from build123d import *

# Parameters (mm, degrees)
EXTRUDE_1_DEPTH     = 16
CUT_EXTRUDE_1_DEPTH = 50
EXTRUDE_2_DEPTH     = 28.5
SKETCH_4_R          = 4.5
CUT_EXTRUDE_2_DEPTH = 28.5


with BuildPart() as part:
    # 草图1 → 凸台-拉伸1 (new, symmetric)
    with BuildSketch(Plane.XY):
        with BuildLine():
            Line((-17, 0), (-17, -66.86388681))
            Line((-17, -66.86388681), (-20.5, -66.86388681))
            Line((-20.5, -66.86388681), (-20.5, 0))
            ThreePointArc((-20.5, 0), (0, 20.5), (20.5, 0))
            Line((20.5, 0), (20.5, -66.86388681))
            Line((20.5, -66.86388681), (17, -66.86388681))
            Line((17, -66.86388681), (17, 0))
            ThreePointArc((17, 0), (0, 17), (-17, 0))
        make_face()
    extrude(amount=EXTRUDE_1_DEPTH, both=True)

    # 草图2 → 切除-拉伸1 (cut, symmetric)
    with BuildSketch(Plane(origin=(0, 0, 0), x_dir=(0, 0, -1), z_dir=(1, 0, 0))):
        Polygon((16, -42.748653355), (-16, -38.251346645), (-16, -66.86388681), (16, -66.86388681), align=None)
    extrude(amount=CUT_EXTRUDE_1_DEPTH, both=True, mode=Mode.SUBTRACT)

    # 草图3 → 凸台-拉伸2 (add)
    with BuildSketch(Plane.ZY.offset(20.5)):
        Polygon((-16, -42.748653355), (16, -38.251346645), (16, -34.716950141), (-16, -39.214256851), align=None)
    extrude_2 = extrude(amount=EXTRUDE_2_DEPTH)

    # 镜向1: 凸台-拉伸2 across plane
    add(extrude_2.mirror(Plane(origin=(0, 0, 0), x_dir=(0, 0, 1), z_dir=(1, 0, 0))))

    # 草图4 → 切除-拉伸2 (cut)
    with BuildSketch(Plane(origin=(0, -36.249611102, 5.094550602), x_dir=(1, 0, 0), z_dir=(0, 0.9902680687415715, -0.13917310096005808))):
        with Locations(Location((40.5, 5.144617667, 0), (0, 0, 270))):
            Circle(SKETCH_4_R)
        with BuildLine():
            Line((-36, 7.644617667), (-36, 2.644617667))
            ThreePointArc((-36, 2.644617667), (-40.5, -1.855382333), (-45, 2.644617667))
            Line((-45, 2.644617667), (-45, 7.644617667))
            ThreePointArc((-45, 7.644617667), (-40.5, 12.144617667), (-36, 7.644617667))
        make_face()
    extrude(amount=-CUT_EXTRUDE_2_DEPTH, mode=Mode.SUBTRACT)


solid = part.part
Input: part model. Units: mm. Frame: model coordinates. A direction names the side the tool comes from. Coordinates: 2 decimals unless noted, no trailing zeros. Order: outer loops, then holes, each group sorted by start corner. A loop starts at its lowest first (then second) coordinate and runs counter-clockwise, first axis right, second up. Notation, with made-up numbers: M 51.5,51 L 109.5,51 A35 ccw 109.5,86 Z; hole C 55,-21 d10. An arc over 180 degrees is marked long. Answer in a Markdown table with one row per item.
(1) Contact query for flat-ended pins moving along their axis: pin 1 Ø3 at (y, z) = (-32, -12) entering from -X; pin 2 Ø12 at (y, z) = (13.5, 0) entering from +X; pin 3 Ø5 at (x, z) = (26, -13) entering from +Y. Output: stop coordinate, or through.
Numbers:
| item | result |
|---|---|
| pin 1 | stops at x = -20.5 |
| pin 2 | stops at x = 19.08 |
| pin 3 | stops at y = -38.44 |
(2) Section query C-C, the plane z = 13.5. Output: boundary loops of the cut face in (x, y), plus the area to 3 significant figures.
Numbers:
| item | result |
|---|---|
| outline | M -49,-38.6 L -17,-38.6 L -17,0 A17 cw 17,0 L 17,-38.6 L 49,-38.6 L 49,-35.07 L 20.5,-35.07 L 20.5,0 A20.5 ccw -20.5,0 L -20.5,-35.07 L -49,-35.07 Z |
| area | 678 mm^2 |
(3) Section query A-A, the plane y = -7. Output: boundary loops of the cut face in (x, z), plus the area to 3 significant figures.
Numbers:
| item | result |
|---|---|
| outline | M -20.5,-16 L -17,-16 L -17,16 L -20.5,16 Z; M 17,-16 L 20.5,-16 L 20.5,16 L 17,16 Z |
| area | 224 mm^2 |
(4) Section query D-D, the plane x = 31. Output: boundary loops of the cut face in (y, z).
Numbers:
| item | result |
|---|---|
| outline | M -42.75,-16 L -39.21,-16 L -34.72,16 L -38.25,16 Z |
(5) Section query B-B, the plane x = 42.5. Output: boundary loops of the cut face in (y, z).
Numbers:
| item | result |
|---|---|
| outline | M -42.75,-16 L -39.21,-16 L -37.53,-3.99 L -40.99,-3.5 Z; M -39.87,4.48 L -36.4,3.99 L -34.72,16 L -38.25,16 Z |
(6) Material intervals for line 1 (X direction, y = -27, z = -8); line 2 (X direction, y = 12, z = 2); line 3 (Y direction, x = -21.5, z = 9), sorted ascending. Write a range as [from, to].
Numbers:
| item | result |
|---|---|
| line 1 | x = [-20.5, -17], [17, 20.5] |
| line 2 | x = [-16.62, -12.04], [12.04, 16.62] |
| line 3 | y = [-39.24, -35.7] |
(7) Access query for faces 1 (the flat face through (-36, -39, 0)), 2 (the flat face through (-34.55, -36.934, 0.224)), 3 (the flat face through (-17, -21, 0)), 4 (the flat face through (34.55, -36.934, 0.224)). Directions: +Z, -Z, +X, -X, +Y, -Y. A direction counts if a zero-diameter tool reaches every point of the face in a straight line with its end or side. Return the directions, or none.
Numbers:
| item | result |
|---|---|
| face 1 | +Y, -Y |
| face 2 | -Z, -X, +Y |
| face 3 | +Z, -Z, -Y |
| face 4 | -Z, +X, +Y |
